The model under review builds one solid part; all positions refer to its coordinate system, in mm. Coordinates: 2 decimals unless noted, no trailing zeros. Loops run counter-clockwise (first coordinate to the right, second up) from the corner with the lowest first, then second, coordinate; pieces in that order, holes last. Notation, with made-up numbers: (19.25, 46.25) - (42.25, 46.25) arc R30 ccw to (42.25, 69.25) - close; hole circle Ø8 at (54.25, -6.75). An arc over 180 degrees is marked (long way). One line per item, written item: value. Start each with the question number.
1. Insertion check: P1, Ø1, axis at x = -27.5, z = 0.5, coming from the +Y side; P2, Ø0.6, axis at x = 28, z = 1.5, coming from the -Y side; P3, Ø1, axis at x = 28, z = 1, coming from the -Y side. Each pin has a flat end and moves straight along its axis. Give the tip position at first contact, or say it passes through.
2. We need section C-C, the plane x = 3.5. Give the boundary of the cut face in (y, z), then the cut area to 3 significant figures.
3. To check wall thickness, follow line 1 (X direction, y = -16.5, z = 0.8); line 2 (Y direction, x = 33.5, z = 0.7); line 3 (Y direction, x = -1.5, z = 0.95). State the ranges of each line that lie inside material, in increasing order.
4. Mouldability with a two-part tool opening along X and no side actions: class faces 1 (the face through (-1, 1, 0)), 2 (the face through (34.423, -41.774, 1.014)), 3 (the face through (0.605, 59.497, 0.986)) as +X half, -X half, draft (parallel to the pull), parting line (faces both ways), or undercut.
5. We need section D-D, the plane z = 1.1. Count the separate pieces of the cut face and the enclosed holes in it, then the cut area to 3 significant figures.
6. We need section B-B, the plane x = -33.5. Give the boundary of the cut face in (y, z).
7. We need section A-A, the plane y = -40. Give the boundary of the cut face in (x, z).
from build123d import *

# Parameters (mm, degrees)
SKIZZE1_R                       = 59.5
AUFSATZ_LINEAR_AUSTRAGEN1_DEPTH = 2
SKIZZE3_R                       = 2
SKIZZE3_W                       = 2.2
SKIZZE3_H                       = 37
SKIZZE3_H_2                     = 17
SKIZZE3_H_3                     = 5.5
SKIZZE3_W_2                     = 30.2
SKIZZE3_H_4                     = 2.2
SKIZZE3_W_3                     = 20
SKIZZE3_H_5                     = 88.994381846
SCHNITT_LINEAR_AUSTRAGEN7_DEPTH = 2


with BuildPart() as part:
    # Skizze1 → Aufsatz-Linear austragen1 (new body)
    with BuildSketch(Plane.XY):
        Circle(SKIZZE1_R)
    extrude(amount=AUFSATZ_LINEAR_AUSTRAGEN1_DEPTH)

    # Skizze3 → Schnitt-Linear austragen7 (cut)
    with BuildSketch(Plane.XY.offset(2)):
        with Locations((-33.5, 40)):
            Circle(SKIZZE3_R)
        with Locations((33.5, 40)):
            Circle(SKIZZE3_R)
        with Locations((33.5, -40)):
            Circle(SKIZZE3_R)
        with Locations((-33.5, -40)):
            Circle(SKIZZE3_R)
        with Locations((-27.6, -0.21138397)):
            Rectangle(SKIZZE3_W, SKIZZE3_H)
        with Locations((27.6, -0.21138397)):
            Rectangle(SKIZZE3_W, SKIZZE3_H)
        with Locations((-27.6, 40.120629313)):
            Rectangle(SKIZZE3_W, SKIZZE3_H_2)
        with Locations((27.6, 40.120629313)):
            Rectangle(SKIZZE3_W, SKIZZE3_H_2)
        with Locations((-27.6, -32.46138397)):
            Rectangle(SKIZZE3_W, SKIZZE3_H_3)
        with Locations((27.6, -32.46138397)):
            Rectangle(SKIZZE3_W, SKIZZE3_H_3)
        with Locations((0, 47.9)):
            Rectangle(SKIZZE3_W_2, SKIZZE3_H_4)
        with Locations((49.5, 0)):
            Rectangle(SKIZZE3_W_3, SKIZZE3_H_5)
        with Locations((-49.5, 0)):
            Rectangle(SKIZZE3_W_3, SKIZZE3_H_5)
    extrude(amount=-SCHNITT_LINEAR_AUSTRAGEN7_DEPTH, mode=Mode.SUBTRACT)


solid = part.part
Findings below:
1. P1: y = 53.02
1. P2: y = -52.66
1. P3: y = -52.76
2. outline: (-59.4, 0) - (46.8, 0) - (46.8, 2) - (-59.4, 2) - close; (49, 0) - (59.4, 0) - (59.4, 2) - (49, 2) - close
2. area: 233 mm2
3. line 1: -39.5 to -28.7, -26.5 to 26.5, 28.7 to 39.5
3. line 2: -49.17 to -42, -38 to 38, 42 to 49.17
3. line 3: -59.48 to 46.8, 49 to 59.48
4. face 1: draft
4. face 2: undercut
4. face 3: parting line
5. separate pieces: 1
5. enclosed holes: 11
5. area: 8,280 mm2
6. outline: (-49.17, 0) - (-42, 0) - (-42, 2) - (-49.17, 2) - close; (-38, 0) - (38, 0) - (38, 2) - (-38, 2) - close; (42, 0) - (49.17, 0) - (49.17, 2) - (42, 2) - close
7. outline: (-39.5, 0) - (-35.5, 0) - (-35.5, 2) - (-39.5, 2) - close; (-31.5, 0) - (31.5, 0) - (31.5, 2) - (-31.5, 2) - close; (35.5, 0) - (39.5, 0) - (39.5, 2) - (35.5, 2) - close
